```python
from build123d import *

# Parameters (mm, degrees)
F1_DEPTH    = 50
F2_T1_DEPTH = 509.1229182759
F3_T        = -2


# Not quite as in the source:
# - a fillet or chamfer that OpenCascade refuses, or shapes differently, is made with other operations: its cross-section is extruded or revolved along the edge and cut away or added


with BuildPart() as f1:
    # F0 (on Front) → F1 (new body, symmetric)
    with BuildSketch(Plane.XZ):
        with BuildLine():
            Line((50, -37.5), (50, 37.5))
            Line((50, 37.5), (25, 37.5))
            ThreePointArc((25, 37.5), (0, 12.5), (-25, 37.5))
            Line((-25, 37.5), (-50, 37.5))
            Line((-50, 37.5), (-50, -37.5))
            Line((-50, -37.5), (50, -37.5))
        make_face()
    extrude(amount=F1_DEPTH, both=True)

    # F2: fillet of radius 100 on 1 edges, made by hand

    # F2_s2 → F2_t1 (cut)
    with BuildSketch(Plane.YZ.offset(-217.061459138)):
        with BuildLine():
            ThreePointArc((-50, -37.5), (-14.4126599144, 16.5569415042), (46.8245836552, 37.5))
            Line((46.8245836552, 37.5), (-50, 37.5))
            Line((-50, 37.5), (-50, -37.5))
        make_face()
    extrude(amount=F2_T1_DEPTH, mode=Mode.SUBTRACT)

    # F3
    f3_openings = [f1.faces().sort_by_distance(p)[0] for p in [
        (0, 50, -4.049992),
        (0, 0, -37.5),
    ]]
    offset(amount=F3_T, openings=f3_openings, kind=Kind.INTERSECTION)


solid = f1.part
```
Check sheet for the modelled part. Datum: model origin and axes. Units: mm. A direction names the side the tool comes from. Give positions to 0.01 mm unless a question says otherwise; leave off trailing zeros. Order: outer loops, then holes, each group sorted by start corner. A loop starts at its lowest first (then second) coordinate and runs counter-clockwise, first axis right, second up. Notation, with made-up numbers: M -27,69 L 4,69 A15 cw 4,79 Z; hole C 78,25.25 d4. An arc over 180 degrees is marked long. Answer in a Markdown table with one row per item. Add a question column.
Q1. Release check for a two-part mould opening along X. For faces 1 (the flat face through (-48.4, -22.5, -37.5)), 2 (the flat face through (-50, 10, -8)), 3 (the cylindrical face through (-0.672, -24.256, 4.966)) record: released by +X, released by -X, zero draft, split by the parting line, or undercut.
Q2. Access from +Z, -Z, +X, -X, +Y, -Y to the whole of each face (thin tool, end or side, straight path). Record for faces 4 (the flat face through (38, 48, 35.5)), 5 (the flat face through (-19, 50, 20)).
Q3. Sectioned sample at B-B, the plane z = 2.5. Record the boundary of the cut face in (x, y), and give its area (3 significant figures).
Q4. Sectioned sample at A-A, the plane x = 0. Record the boundary of the cut face in (y, z), and give its area (3 significant figures).
Q5. Sectioned sample at C-C, the plane y = 16.5. Record the boundary of the cut face in (x, z), and give its area (3 significant figures).
Q6. Thickness scan on L1, parallel to X at y = 35, z = -26; L2, parallel to X at y = 38.5, z = 33; L3, parallel to Z at x = -1, y = 33. Record the ranges inside material, lowest first.
Q7. Gauge pin test, flat ends, axial feed: pin 1 Ø3.5 at (x, y) = (-36.5, 48) entering from -Z; pin 2 Ø3 at (x, y) = (1.5, -18) entering from -Z; pin 3 Ø2 at (x, z) = (-11, -28) entering from +Y. Record the tip position at first contact, or that the pin passes through.
Q8. Sectioned sample at D-D, the plane y = -13.5. Record the boundary of the cut face in (x, z).
Verdict:
| question | item | result |
|---|---|---|
| 1 | face 1 | zero draft |
| 1 | face 2 | released by -X |
| 1 | face 3 | undercut |
| 2 | face 4 | -Z, +Y |
| 2 | face 5 | +Z, -Z, +X, -X, +Y |
| 3 | outline | M -50,-29.17 L 50,-29.17 L 50,50 L 48,50 L 48,-26.52 L -48,-26.52 L -48,50 L -50,50 Z |
| 3 | area | 571 mm² |
| 4 | outline | M -50,-37.5 L -47.93,-37.5 A98 cw -18.56,10.5 L 50,10.5 L 50,12.5 L -19.32,12.5 A100 ccw Z |
| 4 | area | 254 mm² |
| 5 | outline | M -50,-37.5 L -48,-37.5 L -48,30.69 L -26.13,30.69 A27 ccw 26.13,30.69 L 48,30.69 L 48,-37.5 L 50,-37.5 L 50,32.79 L 24.55,32.79 A25 cw -24.55,32.79 L -50,32.79 Z |
| 5 | area | 516 mm² |
| 6 | L1 | -50 to -48, 48 to 50 |
| 6 | L2 | -50 to -48, -26.62 to -24.59, 24.59 to 26.62, 48 to 50 |
| 6 | L3 | 10.52 to 12.52 |
| 7 | pin 1 | z = 35.5 |
| 7 | pin 2 | z = 9.65 |
| 7 | pin 3 | y = -44.52 |
| 8 | outline | M -50,-37.5 L -48,-37.5 L -48,14.73 L -14.51,14.73 A27 ccw 14.51,14.73 L 48,14.73 L 48,-37.5 L 50,-37.5 L 50,17.26 L 14.67,17.26 A25 cw -14.67,17.26 L -50,17.26 Z |
